Work out the finished part from the listing and answer in its coordinate system (mm). Face numbers are marked on the shaded views. A direction names the side the tool comes from. Round coordinates to 2 decimals unless told otherwise and drop trailing zeros. Loops run counter-clockwise (first coordinate to the right, second up) from the corner with the lowest first, then second, coordinate; pieces in that order, holes last. Notation, with made-up numbers: (72.25, 30) - (101.25, 30) arc R28 cw to (101.25, 58) - close; hole circle Ø3 at (66.25, 70). An arc over 180 degrees is marked (long way). Answer as CSV lines item,"result". Start each with the question number.
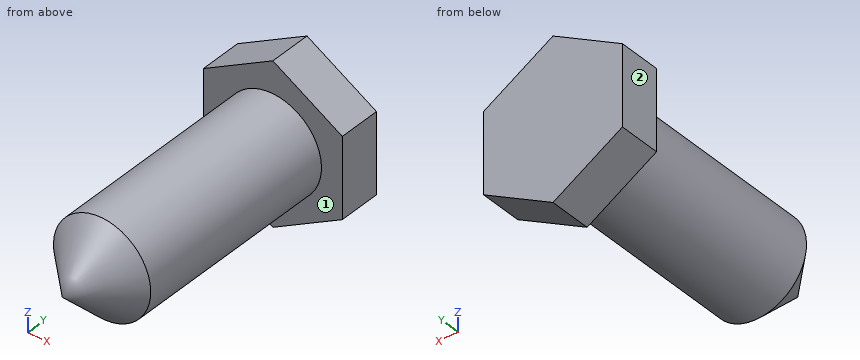
Autodesk Inventor part; units mm, degrees
ref_plane "YZ Plane" through (0, 0, 0) normal (1, 0, 0) x (0, 1, 0)
ref_plane "XZ Plane" through (0, 0, 0) normal (0, 1, 0) x (-1, 0, 0)
ref_plane "XY Plane" through (0, 0, 0) normal (0, 0, 1) x (1, 0, 0)
sketch "Sketch1" plane through (0, 0, 0) normal (1, 0, 0) x (0, 1, 0)
  line L0 (0, 0) -> (18.5, 0)
  line L1 (18.5, 0) -> (18.5, 3.5)
  line L2 (18.5, 3.5) -> (3.5, 3.5)
  line L3 (3.5, 3.5) -> (0, 0)
  dimension "d0" = 135
  dimension "d1" = 3.5
  dimension "d2" = 18.5
revolve "Revolution1" add sketch "Sketch1" angle 360 about axis through (0, 0, 0) along (0, 1, 0)
thread "Thread1"
sketch "Sketch2" plane through (0, 18.5, 0) normal (0, 1, 0) x (1, 0, 0)
  circle A0 centre (0, 0) radius 5 construction
  line L0 (-5, -2.8868) -> (-5, 2.8868)
  line L1 (-5, 2.8868) -> (0, 5.7735)
  line L2 (0, 5.7735) -> (5, 2.8868)
  line L3 (5, 2.8868) -> (5, -2.8868)
  line L4 (5, -2.8868) -> (0, -5.7735)
  line L5 (0, -5.7735) -> (-5, -2.8868)
  dimension "d6" = 10
  dimension "d7" = 120
extrude "Extrusion1" add sketch "Sketch2" along normal blind 3
properties part number "side bolt"
Item 1: Which of the six approach directions +Z, -Z, +X, -X, +Y, -Y give full straight-line access (tool end or side, diameter ignored) to the marked faces 1 and 2?
Item 2: Section A-A, the plane y = 1.75 is taken. Give the vertices of the cut face in (x, z).
Item 3: Section D-D, the plane y = 6.25 is taken. Give the vertices of the cut face in (x, z), and give its area (3 significant figures).
Item 4: Find the intervals of material crossed by L1, parallel to Y at x = -2.25, z = 3.5; L2, parallel to X at y = 3.25, z = 0.5; L3, parallel to X at y = 19.25, z = 4.75, in increasing order.
Item 5: Section C-C, the plane y = 19.5 is taken. Give the vertices of the cut face in (x, z).
Item 6: Flat-ended cylindrical pins translate along their axes: pin 1 Ø3 at (x, z) = (-1.5, 1.5) entering from -Y; pin 2 Ø5 at (x, y) = (2.5, 5.5) entering from +Z; pin 3 Ø1 at (y, z) = (13, -0.5) entering from +X. Find the tip coordinate at first contact, or state that the pin passes through.
Item 7: Section B-B, the plane z = 4.75 is taken. Give the vertices of the cut face in (x, y).
Answer:
1,face 1,"-Y"
1,face 2,"+Z, -Z, -X, +Y, -Y"
2,outline,"circle Ø3.5 at (0, 0)"
3,outline,"circle Ø7 at (0, 0)"
3,area,"38.5 mm²"
4,L1,"y = 18.5 to 21.5"
4,L2,"x = -3.21 to 3.21"
4,L3,"x = -1.77 to 1.77"
5,outline,"(-5, -2.89) - (0, -5.77) - (5, -2.89) - (5, 2.89) - (0, 5.77) - (-5, 2.89) - close"
6,pin 1,"stops at y = 0.62"
6,pin 2,"stops at z = 3.5"
6,pin 3,"stops at x = 3.5"
7,outline,"(-1.77, 18.5) - (1.77, 18.5) - (1.77, 21.5) - (-1.77, 21.5) - close"
